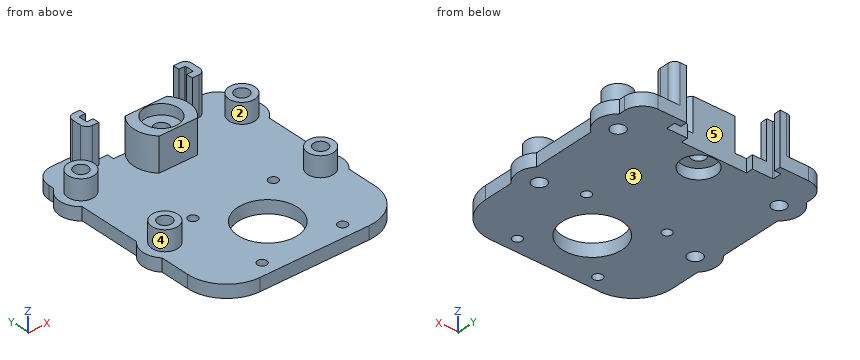
from build123d import *

# Parameters (mm, degrees)
SKETCH_1_R      = 2.7
SKETCH_1_R_2    = 6.6
SKETCH_1_R_3    = 1.8
SKETCH_1_R_4    = 11.5
EXTRUDE_1_DEPTH = 5
EXTRUDE_START   = 4
EXTRUDE_3_DEPTH = 16
FILLET_1_R      = 2.5
FILLET_2_R      = 0.3
SKETCH_9_R      = 5
SKETCH_9_R_2    = 2.7
EXTRUDE_4_DEPTH = 7.7
SKETCH_1_5_R    = 6.6
SKETCH_1_5_R_2  = 2.7
EXTRUDE_5_DEPTH = 10
EXTRUDE_START_2 = 14
SKETCH_1_6_R    = 6.6
EXTRUDE_6_DEPTH = 4


with BuildPart() as part:
    # 草图1 → 凸台-拉伸1 (new body)
    with BuildSketch(Plane.XY):
        with BuildLine():
            ThreePointArc((-29, 43.7), (-33.949747468, 41.649747468), (-36, 36.7))
            Line((-36, 36.7), (-36, 34.472597587))
            ThreePointArc((-36, 34.472597587), (-39.1, 28.1), (-36, 21.727402413))
            Line((-36, 21.727402413), (-36, -2.565019616))
            ThreePointArc((-36, -2.565019616), (-38.3, -8.3), (-36, -14.034980384))
            Line((-36, -14.034980384), (-36, -25.5))
            ThreePointArc((-36, -25.5), (-31.606601718, -36.106601718), (-21, -40.5))
            Line((-21, -40.5), (21, -40.5))
            ThreePointArc((21, -40.5), (31.606601718, -36.106601718), (36, -25.5))
            Line((36, -25.5), (36, -14.034980384))
            ThreePointArc((36, -14.034980384), (38.3, -8.3), (36, -2.565019616))
            Line((36, -2.565019616), (36, 21.727402413))
            ThreePointArc((36, 21.727402413), (39.1, 28.1), (36, 34.472597587))
            Line((36, 34.472597587), (36, 36.7))
            ThreePointArc((36, 36.7), (33.949747468, 41.649747468), (29, 43.7))
            Line((29, 43.7), (18, 43.7))
            Line((18, 43.7), (18, 41.2))
            Line((18, 41.2), (20.5, 41.2))
            Line((20.5, 41.2), (20.5, 37.7))
            Line((20.5, 37.7), (12.5, 37.7))
            Line((12.5, 37.7), (12.5, 35))
            Line((12.5, 35), (-12.5, 35))
            Line((-12.5, 35), (-12.5, 37.7))
            Line((-12.5, 37.7), (-20.5, 37.7))
            Line((-20.5, 37.7), (-20.5, 41.2))
            Line((-20.5, 41.2), (-18, 41.2))
            Line((-18, 41.2), (-18, 43.7))
            Line((-18, 43.7), (-29, 43.7))
        make_face()
        with Locations((-31, 28.1)):
            Circle(SKETCH_1_R, mode=Mode.SUBTRACT)
        with Locations((-30, -8.3)):
            Circle(SKETCH_1_R, mode=Mode.SUBTRACT)
        with Locations((0, 28.1)):
            Circle(SKETCH_1_R_2, mode=Mode.SUBTRACT)
        with Locations((15.5, -4)):
            Circle(SKETCH_1_R_3, mode=Mode.SUBTRACT)
        with Locations((0, -19.5)):
            Circle(SKETCH_1_R_4, mode=Mode.SUBTRACT)
        with Locations((15.5, -35)):
            Circle(SKETCH_1_R_3, mode=Mode.SUBTRACT)
        with Locations((-15.5, -35)):
            Circle(SKETCH_1_R_3, mode=Mode.SUBTRACT)
        with Locations((-15.5, -4)):
            Circle(SKETCH_1_R_3, mode=Mode.SUBTRACT)
        with Locations((30, -8.3)):
            Circle(SKETCH_1_R, mode=Mode.SUBTRACT)
        with Locations((31, 28.1)):
            Circle(SKETCH_1_R, mode=Mode.SUBTRACT)
    extrude(amount=EXTRUDE_1_DEPTH)

    # 草图1<4> → 凸台-拉伸3 (add)
    with BuildSketch(Plane.XY.offset(EXTRUDE_START)):
        Polygon((-18, 43.7), (-23, 43.7), (-23, 35.2), (-18, 35.2), (-18, 37.7), (-20.5, 37.7), (-20.5, 41.2), (-18, 41.2), align=None)
        Polygon((20.5, 37.7), (18, 37.7), (18, 35.2), (23, 35.2), (23, 43.7), (18, 43.7), (18, 41.2), (20.5, 41.2), align=None)
    extrude(amount=EXTRUDE_3_DEPTH)

    # 圆角1
    fillet_1_edges = [part.edges().sort_by_distance(p)[0] for p in [
        (-23, 35.2, 12.5),
        (-23, 43.7, 12.5),
        (23, 35.2, 12.5),
        (23, 43.7, 12.5),
    ]]
    fillet(fillet_1_edges, radius=FILLET_1_R)

    # 圆角2
    fillet_2_edges = [part.edges().sort_by_distance(p)[0] for p in [
        (20.5, 37.7, 10),
        (20.5, 41.2, 10),
        (-20.5, 41.2, 10),
        (-20.5, 37.7, 10),
    ]]
    fillet(fillet_2_edges, radius=FILLET_2_R)

    # 草图9 → 凸台-拉伸4 (add)
    # profile 1 of 4: a face of its own
    with BuildSketch(Plane.XY.offset(5)):
        with Locations(Location((-31, 28.1, 0), (0, 0, 180))):
            Circle(SKETCH_9_R)
        with Locations((-31, 28.1)):
            Circle(SKETCH_9_R_2, mode=Mode.SUBTRACT)
    # profile 2 of 4: a face of its own
    with BuildSketch(Plane.XY.offset(5)):
        with Locations(Location((-30, -8.3, 0), (0, 0, 180))):
            Circle(SKETCH_9_R)
        with Locations((-30, -8.3)):
            Circle(SKETCH_9_R_2, mode=Mode.SUBTRACT)
    # profile 3 of 4: a face of its own
    with BuildSketch(Plane.XY.offset(5)):
        with Locations(Location((30, -8.3, 0), (0, 0, 180))):
            Circle(SKETCH_9_R)
        with Locations(Location((30, -8.3, 0), (0, 0, 180))):
            Circle(SKETCH_9_R_2, mode=Mode.SUBTRACT)
    # profile 4 of 4: a face of its own
    with BuildSketch(Plane.XY.offset(5)):
        with Locations(Location((31, 28.1, 0), (0, 0, 180))):
            Circle(SKETCH_9_R)
        with Locations(Location((31, 28.1, 0), (0, 0, 180))):
            Circle(SKETCH_9_R_2, mode=Mode.SUBTRACT)
    extrude(amount=EXTRUDE_4_DEPTH)

    # 草图1<5> → 凸台-拉伸5 (add)
    # profile 1 of 2: a face of its own
    with BuildSketch(Plane.XY.offset(EXTRUDE_START)):
        with BuildLine():
            Line((8.04673847, 35), (-8.04673847, 35))
            ThreePointArc((-8.04673847, 35), (-10.589117274, 27.619796539), (-7.389181281, 20.5))
            Line((-7.389181281, 20.5), (7.389181281, 20.5))
            ThreePointArc((7.389181281, 20.5), (10.589117274, 27.619796539), (8.04673847, 35))
        make_face()
        with Locations((0, 28.1)):
            Circle(SKETCH_1_5_R, mode=Mode.SUBTRACT)
    # profile 2 of 2: a face of its own
    with BuildSketch(Plane.XY.offset(EXTRUDE_START)):
        with Locations((0, 28.1)):
            Circle(SKETCH_1_5_R)
        with Locations((0, 28.1)):
            Circle(SKETCH_1_5_R_2, mode=Mode.SUBTRACT)
    extrude(amount=EXTRUDE_5_DEPTH)

    # 草图1<6> → 凸台-拉伸6 (add)
    with BuildSketch(Plane.XY.offset(EXTRUDE_START_2)):
        with BuildLine():
            Line((8.04673847, 35), (-8.04673847, 35))
            ThreePointArc((-8.04673847, 35), (-10.589117274, 27.619796539), (-7.389181281, 20.5))
            Line((-7.389181281, 20.5), (7.389181281, 20.5))
            ThreePointArc((7.389181281, 20.5), (10.589117274, 27.619796539), (8.04673847, 35))
        make_face()
        with Locations((0, 28.1)):
            Circle(SKETCH_1_6_R, mode=Mode.SUBTRACT)
    extrude(amount=EXTRUDE_6_DEPTH)


solid = part.part
For this review, take the finished solid that the model builds, in its own axes (mm). Face numbers are marked on the shaded views. A direction names the side the tool comes from. Give positions to 0.01 mm unless a question says otherwise; leave off trailing zeros. Order: outer loops, then holes, each group sorted by start corner. A loop starts at its lowest first (then second) coordinate and runs counter-clockwise, first axis right, second up. Notation, with made-up numbers: (0.25, -27) - (29.25, -27) arc R24 cw to (29.25, 2) - close; hole circle Ø2 at (30, -13). An arc over 180 degrees is marked (long way). Answer as a JSON object with one key per item and string values. Group by question number.
Item 1: Clearance check with flat-ended pins moving along their axes: pin 1 Ø3 at (x, y) = (31, -6.5) entering from +Z; pin 2 Ø5 at (x, y) = (0, 28.1) entering from +Z; pin 3 Ø4 at (x, z) = (4.5, 14.5) entering from -Y; pin 4 Ø12 at (x, z) = (-17, 15) entering from -Y. State where each tip first meets the part, or that it passes through.
Item 2: Machinability: for the marked faces 1 and 2, which of the approach directions +Z, -Z, +X, -X, +Y, -Y give a long, thin tool a straight path to every point of the face, cutting with its end or side? Answer none if there is none.
Item 3: Take a section at B-B on x = -15.5. Give the boundary of the cut face in (y, z), and give its area (3 significant figures).
Item 4: Take a section at D-D on y = -10. Give the boundary of the cut face in (x, z), and give its area (3 significant figures).
Item 5: Wall thickness on line 1 along Y through (x, z) = (0, 3.7); line 2 along Y through (x, z) = (-15.5, 2.7); line 3 along Y through (x, z) = (20, 12): over which ranges is each line inside the solid? List them lowest first.
Item 6: Take a section at A-A on y = -19.5. Give the boundary of the cut face in (x, z).
Item 7: Take a section at C-C on z = 2. Give the number of separate pieces and of enclosed holes in the cut face, and give its area (3 significant figures).
Item 8: Draft analysis for pull direction Y (two halves, no side actions). For the marked faces 3, 4 and 5, state which applies: pulls with the +Y half, pulls with the -Y half, needs draft (parallel to the pull), parting line crosses it, or undercut.
Reported:
{
 "1": {"pin 1": "z = 12.7", "pin 2": "through", "pin 3": "y = 20.5", "pin 4": "y = 35.2"},
 "2": {"face 1": "+Z, +X, -X, -Y", "face 2": "+Z"},
 "3": {"outline": "(-40.5, 0) - (-36.8, 0) - (-36.8, 5) - (-40.5, 5) - close; (-33.2, 0) - (-5.8, 0) - (-5.8, 5) - (-33.2, 5) - close; (-2.2, 0) - (37.7, 0) - (37.7, 5) - (-2.2, 5) - close", "area": "355 mm^2"},
 "4": {"outline": "(-38.12, 0) - (-32.1, 0) - (-32.1, 12.7) - (-34.7, 12.7) - (-34.7, 5) - (-38.12, 5) - close; (-27.9, 0) - (-6.48, 0) - (-6.48, 5) - (-25.3, 5) - (-25.3, 12.7) - (-27.9, 12.7) - close; (6.48, 0) - (27.9, 0) - (27.9, 12.7) - (25.3, 12.7) - (25.3, 5) - (6.48, 5) - close; (32.1, 0) - (38.12, 0) - (38.12, 5) - (34.7, 5) - (34.7, 12.7) - (32.1, 12.7) - close", "area": "355 mm^2"},
 "5": {"line 1": "-40.5 to -31, -8 to 21.5, 34.7 to 35", "line 2": "-40.5 to -36.8, -33.2 to -5.8, -2.2 to 37.7", "line 3": "35.2 to 37.7, 41.2 to 43.7"},
 "6": {"outline": "(-36, 0) - (-11.5, 0) - (-11.5, 5) - (-36, 5) - close; (11.5, 0) - (36, 0) - (36, 5) - (11.5, 5) - close"},
 "7": {"separate pieces": "1", "enclosed holes": "10", "area": "5,050 mm^2"},
 "8": {"face 3": "needs draft", "face 4": "undercut", "face 5": "pulls with the +Y half"}
}
